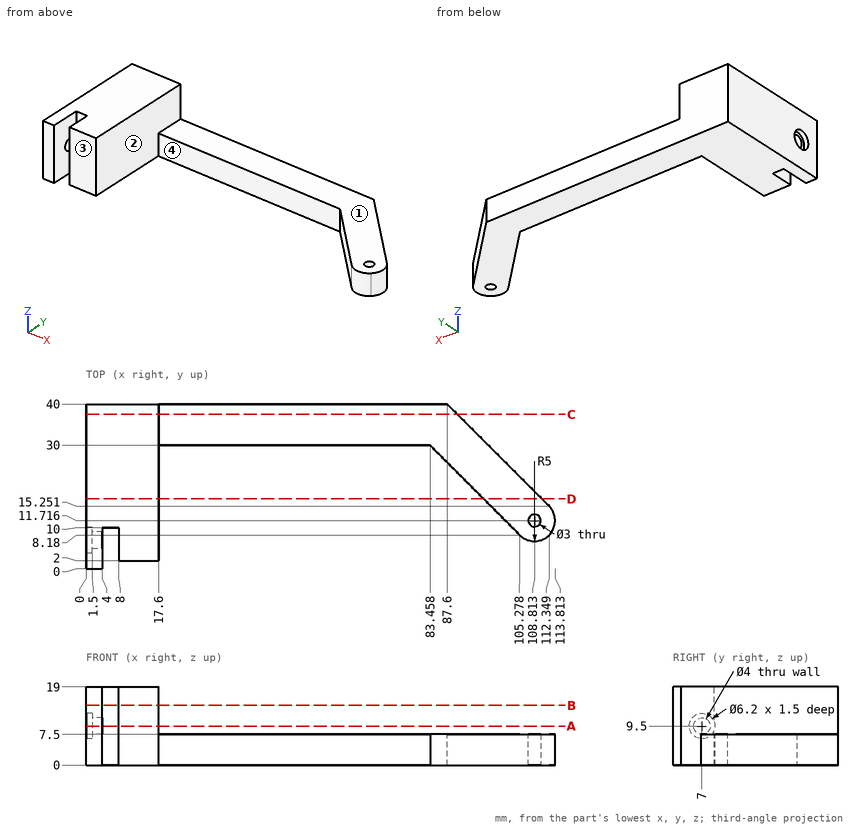
Answer from the drawing. Dimensions are ordinates in mm from the lowest x, y and z of the part. A direction names the side the tool comes from. Give positions to 0.01 mm unless a question says otherwise; leave off trailing zeros. Order: outer loops, then holes, each group sorted by start corner. A loop starts at its lowest first (then second) coordinate and runs counter-clockwise, first axis right, second up. Notation, with made-up numbers: (10.25, -30) - (34.25, -30) arc R24 cw to (34.25, 0) - close; hole circle Ø4 at (-37, -33). An arc over 180 degrees is marked (long way). One line per item, written item: value. Start each with the question number.
1) A cutting plane is placed at B-B on z = 14.5. Give the vertices of the cut face in (x, y).
2) A cutting plane is placed at D-D on y = 17. Give the vertices of the cut face in (x, z).
3) A cutting plane is placed at C-C on y = 37.5. Give the vertices of the cut face in (x, z).
4) A tool of negligible diameter and unlimited length cuts with its end or side. For the marked faces 1, 2, 3 and 4, from which of +Z, -Z, +X, -X, +Y, -Y can it reach the whole face along a straight path? Write none if from no direction.
5) A cutting plane is placed at A-A on z = 9.5. Give the vertices of the cut face in (x, y).
6) Given pin 1 Ø5 at (x, z) = (49.5, 8) entering from -Y; pin 2 Ø9.5 at (y, z) = (27, 7.5) entering from +X; pin 3 Ø8 at (x, z) = (43.5, 9) entering from +Y; pin 4 Ø7.5 at (x, z) = (12.5, 8) entering from -Y, each flat-ended and moving along its own axis, determine where each tip first touches the part or whether it passes through.
7) Find the intervals of material crossed by L1, parallel to Z at x = 1, y = 7; L2, parallel to X at y = 3, z = 3.75; L3, parallel to X at y = 13, z = 10.25, in increasing order.
Answer sheet:
1. outline: (0, 0) - (4, 0) - (4, 10) - (8, 10) - (8, 2) - (17.6, 2) - (17.6, 40) - (0, 40) - close
2. outline: (0, 0) - (17.6, 0) - (17.6, 19) - (0, 19) - close; (96.46, 0) - (110.6, 0) - (110.6, 7.5) - (96.46, 7.5) - close
3. outline: (0, 0) - (90.1, 0) - (90.1, 7.5) - (17.6, 7.5) - (17.6, 19) - (0, 19) - close
4. face 1: +Z, +X, +Y, -Y
4. face 2: +Z, -Y
4. face 3: +Z, -Z, +X, -Y
4. face 4: +Z, -Z, -Y
5. outline: (0, 0) - (4, 0) - (4, 5) - (1.5, 5) - (1.5, 3.9) - (0, 3.9) - close; (0, 10.1) - (1.5, 10.1) - (1.5, 9) - (4, 9) - (4, 10) - (8, 10) - (8, 2) - (17.6, 2) - (17.6, 40) - (0, 40) - close
6. pin 1: stops at y = 30
6. pin 2: stops at x = 105.35
6. pin 3: stops at y = 40
6. pin 4: stops at y = 2
7. L1: z = 0 to 6.4, 12.6 to 19
7. L2: x = 0 to 4, 8 to 17.6
7. L3: x = 0 to 17.6
